```python
from build123d import *

# Parameters (mm, degrees)
SKETCH_1_R          = 8
EXTRUDE_1_DEPTH     = 0.65
EXTRUDE_START       = 0.65
SKETCH_2_R          = 6.12
SKETCH_2_R_2        = 5.1
EXTRUDE_2_DEPTH     = 0.85
CUT_EXTRUDE_START   = 0.65
SKETCH_3_R          = 5.1
CUT_EXTRUDE_1_DEPTH = 0.01
CUT_EXTRUDE_2_DEPTH = 0.64
CHAMFER_1_SIZE      = 0.3


with BuildPart() as part:
    # 草图1 → 凸台-拉伸1 (new body)
    with BuildSketch(Plane.XY):
        Circle(SKETCH_1_R)
    extrude(amount=EXTRUDE_1_DEPTH)

    # 草图2 → 凸台-拉伸2 (add)
    with BuildSketch(Plane.XY.offset(EXTRUDE_START)):
        Circle(SKETCH_2_R)
        Circle(SKETCH_2_R_2, mode=Mode.SUBTRACT)
    extrude(amount=EXTRUDE_2_DEPTH)

    # 草图3 → 切除-拉伸1 (cut)
    with BuildSketch(Plane.XY.offset(CUT_EXTRUDE_START)):
        Circle(SKETCH_3_R)
    extrude(amount=-CUT_EXTRUDE_1_DEPTH, mode=Mode.SUBTRACT)

    # 草图4 → 切除-拉伸2 (cut)
    with BuildSketch(Plane.XY):
        Polygon((3.75, 3.75), (3.75, -3.75), (-3.75, -3.75), (-3.75, 0), (-3.75, 3.75), align=None)
    extrude(amount=CUT_EXTRUDE_2_DEPTH, mode=Mode.SUBTRACT)

    # 倒角1
    chamfer_1_edges = [part.edges().sort_by_distance(p)[0] for p in [
        (-5.1, 0, 1.5),
    ]]
    chamfer(chamfer_1_edges, length=CHAMFER_1_SIZE)


solid = part.part
```
Verification items for the finished model (mm, model axes). A direction names the side the tool comes from. Coordinates: 2 decimals unless noted, no trailing zeros. Loops run counter-clockwise (first coordinate to the right, second up) from the corner with the lowest first, then second, coordinate; pieces in that order, holes last. Notation, with made-up numbers: (14.5, 77) -> (46.5, 77) arc R28 ccw to (46.5, 98) -> close; hole circle Ø8 at (53, -6.5). An arc over 180 degrees is marked (long way). Answer in a Markdown table with one row per item. Add a question column.
1. Access from +Z, -Z, +X, -X, +Y, -Y to the whole of each face (thin tool, end or side, straight path). Record for faces 4 (the face through (4, -4, 1.5)), 5 (the face through (2.4, -4.5, 0.9)).
2. Draft check along Y on faces 1 (the face through (0, -4, 0.64)), 2 (the face through (-1.73, -7.81, 0.32)), 3 (the face through (5, 0, 0)). Enter one of: +Y half, -Y half, draft (parallel to the pull), parting line (faces both ways), or undercut.
3. Material ranges on probe 1 along Y at (x, z) = (0, 0.95); probe 2 along X at (y, z) = (-4.25, 0.9); probe 3 along Z at (x, y) = (-5.25, -4.75), recorded low to high. Write a range as [from, to].
4. Section check A-A, the plane y = 0. Enter the section's corners in (x, z).
5. Depth check by flat-ended pin: P1, Ø0.7, axis at y = -0.5, z = 0.5, coming from the +X side; P2, Ø1, axis at x = -6.5, y = 3.5, coming from the +Z side; P3, Ø0.7, axis at y = 0.5, z = 0.5, coming from the -X side. Enter the tip coordinate at first touch or a pass-through.
6. Section check C-C, the plane z = 0.35. Enter the section's corners in (x, y), then the cut area to 3 significant figures.
7. Section check D-D, the plane x = -7. Enter the section's corners in (y, z), then the cut area to 3 significant figures.
Derived:
| question | item | result |
|---|---|---|
| 1 | face 4 | +Z, +X, -X, +Y, -Y |
| 1 | face 5 | +Z |
| 2 | face 1 | undercut |
| 2 | face 2 | parting line |
| 2 | face 3 | draft |
| 3 | probe 1 | y = [-6.12, -5.1], [5.1, 6.12] |
| 3 | probe 2 | x = [-4.4, -2.82], [2.82, 4.4] |
| 3 | probe 3 | z = [0, 0.65] |
| 4 | outline | (-8, 0) -> (-3.75, 0) -> (-3.75, 0.64) -> (-5.1, 0.64) -> (-5.1, 1.2) -> (-5.4, 1.5) -> (-6.12, 1.5) -> (-6.12, 0.65) -> (-8, 0.65) -> close; (3.75, 0) -> (8, 0) -> (8, 0.65) -> (6.12, 0.65) -> (6.12, 1.5) -> (5.4, 1.5) -> (5.1, 1.2) -> (5.1, 0.64) -> (3.75, 0.64) -> close |
| 5 | P1 | stops at x = 8 |
| 5 | P2 | stops at z = 0.65 |
| 5 | P3 | stops at x = -8 |
| 6 | outline | circle Ø16 at (0, 0); hole (-3.75, -3.75) -> (3.75, -3.75) -> (3.75, 3.75) -> (-3.75, 3.75) -> close |
| 6 | area | 145 mm² |
| 7 | outline | (-3.87, 0) -> (3.87, 0) -> (3.87, 0.65) -> (-3.87, 0.65) -> close |
| 7 | area | 5.03 mm² |
